Work out the finished part from the listing and answer in its coordinate system (mm). A direction names the side the tool comes from. Coordinates: 2 decimals unless noted, no trailing zeros. Order: outer loops, then holes, each group sorted by start corner. A loop starts at its lowest first (then second) coordinate and runs counter-clockwise, first axis right, second up. Notation, with made-up numbers: M -33,54 L 23,54 A34 cw 23,93 Z; hole C 47.5,80.25 d2. An arc over 180 degrees is marked long. Use a Markdown table: item, result. Add a question column.
from build123d import *

# Parameters (mm, degrees)
SKETCH1_W               = 25.4
SKETCH1_H               = 3.175
SKETCH1_W_2             = 1.5875
SKETCH1_H_2             = 1.5875
SKETCH1_W_3             = 7.9375
SKETCH1_H_3             = 2.38125
CUT_EXTRUDE1_DEPTH      = 27.940768363
CUT_EXTRUDE1_DEPTH_BACK = 27.940768363
SKETCH2_W               = 0.79375
SKETCH2_H               = 3.175
SKETCH2_R               = 1.5875
FILLET1_R               = 1.5875
CHAMFER1_SIZE           = 1.5875


with BuildPart() as part:
    # Sketch1 → Revolve1 (revolve)
    with BuildSketch(Plane.XY):
        with Locations((-12.7, 1.5875)):
            Rectangle(SKETCH1_W, SKETCH1_H)
        with Locations((-0.79375, 3.96875)):
            Rectangle(SKETCH1_W_2, SKETCH1_H_2)
        Polygon((0, 3.175), (0, 0), (2.38125, 0), (2.38125, 3.96875), (2.38125, 6.35), (0, 6.35), (0, 4.7625), align=None)
        with Locations((6.35, 5.159375)):
            Rectangle(SKETCH1_W_3, SKETCH1_H_3)
    revolve(axis=Axis((0, 0, 0), (-1, 0, 0)))

    # Sketch2 → Cut-Extrude1 (cut, two sides: drawn at the far end of the back side and taken through both)
    with BuildSketch(Plane(origin=(0, 0, 0), x_dir=(1, 0, 0), z_dir=(0, 1, 0)).offset(-CUT_EXTRUDE1_DEPTH_BACK)):
        with Locations((2.778125, 0)):
            Rectangle(SKETCH2_W, SKETCH2_H)
        with BuildLine():
            Line((3.175, -1.5875), (6.35, -1.5875))
            ThreePointArc((6.35, -1.5875), (4.7625, 0), (6.35, 1.5875))
            Line((6.35, 1.5875), (3.175, 1.5875))
            Line((3.175, 1.5875), (3.175, -1.5875))
        make_face()
        with Locations((6.35, 0)):
            Circle(SKETCH2_R)
        with BuildLine():
            Line((6.35, -1.5875), (10.31875, -1.5875))
            Line((10.31875, -1.5875), (10.31875, 1.5875))
            Line((10.31875, 1.5875), (6.35, 1.5875))
            ThreePointArc((6.35, 1.5875), (7.472532015, 1.122532015), (7.9375, 0))
            ThreePointArc((7.9375, 0), (7.472532015, -1.122532015), (6.35, -1.5875))
        make_face()
    extrude(amount=CUT_EXTRUDE1_DEPTH + CUT_EXTRUDE1_DEPTH_BACK, mode=Mode.SUBTRACT)

    # Fillet1
    fillet1_edges = [part.edges().sort_by_distance(p)[0] for p in [
        (2.38125, -4.89289026, -1.5875),
        (2.38125, 4.89289026, -1.5875),
        (2.38125, -4.89289026, 1.5875),
        (2.38125, 4.89289026, 1.5875),
    ]]
    fillet(fillet1_edges, radius=FILLET1_R - 0.0001)  # a hair under: the kernel refuses the full size

    # Chamfer1
    chamfer1_edges = [part.edges().sort_by_distance(p)[0] for p in [
        (10.31875, 0, 3.96875),
        (10.31875, 0, -3.96875),
    ]]
    chamfer(chamfer1_edges, length=CHAMFER1_SIZE)


solid = part.part
(1) Given P1, Ø6, axis at x = -10.5, y = 3.5, coming from the -Z side; P2, Ø2, axis at x = 8, y = -5, coming from the -Z side; P3, Ø1, axis at y = 2, z = -4.5, coming from the -X side; P4, Ø1.5, axis at x = -11, y = 4, coming from the -Z side, each flat-ended and moving along its own axis, determine where each tip first touches the part or whether it passes through.
(2) A cutting plane is placed at D-D on x = -12. Write down the section's boundary in (y, z) (3 decimals).
(3) The mould has two halves that part along Z. Classify faces 5 (the flat face through (0, 1, -5)), 6 (the cylindrical face through (2.859, 5.013, -1.135)), 7 (the cylindrical face through (-0.78, -3.78, 2.9)): pulls with the +Z half, pulls with the -Z half, needs draft (parallel to the pull), parting line crosses it, or undercut.
(4) Straight lines are drawn through the part: line 1 (X direction, y = -0.5, z = -3.5); line 2 (Z direction, x = 3, y = -1.75); line 3 (X direction, y = -2.75, z = 0.5). For each, find the intervals that lie inside material, in ascending order.
(5) A cutting plane is placed at C-C on z = -1. Write down the section's boundary in (x, y).
(6) A cutting plane is placed at A-A on x = 3.5. Write down the section's boundary in (y, z), plus the area to 3 significant figures.
(7) Which of the six approach directions +Z, -Z, +X, -X, +Y, -Y give full straight-line access (tool end or side, diameter ignored) to faces 1 (the flat face through (-25.4, 0, 0)), 2 (the cylindrical face through (-13.33, -0.69, 3.1)), 3 (the flat face through (7, 5, 1.588)), 4 (the cylindrical face through (5.601, 0.087, -3.968))?
From the geometry:
| question | item | result |
|---|---|---|
| 1 | P1 | stops at z = -3.14 |
| 1 | P2 | stops at z = -4.93 |
| 1 | P3 | stops at x = -1.59 |
| 1 | P4 | passes through |
| 2 | outline | C 0,0 d6.35 |
| 3 | face 5 | needs draft |
| 3 | face 6 | undercut |
| 3 | face 7 | parting line crosses it |
| 4 | line 1 | x = -1.59 to 2.38 |
| 4 | line 2 | z = -6.1 to -3.56, 3.56 to 6.1 |
| 4 | line 3 | x = -25.4 to 2.38 |
| 5 | outline | M -25.4,-3.01 L -1.59,-3.01 L -1.59,-4.66 L 0,-4.66 L 0,-6.27 L 2.74,-6.27 L 2.74,-3.84 L 2.38,-3.84 L 2.38,3.84 L 2.74,3.84 L 2.74,6.27 L 0,6.27 L 0,4.66 L -1.59,4.66 L -1.59,3.01 L -25.4,3.01 Z |
| 6 | outline | M -6.17,-1.52 A6.35 ccw 6.17,-1.52 L 3.67,-1.52 A3.97 cw -3.67,-1.52 Z; M -6.17,1.52 L -3.67,1.52 A3.97 cw 3.67,1.52 L 6.17,1.52 A6.35 ccw Z |
| 6 | area | 62.5 mm2 |
| 7 | face 1 | +Z, -Z, -X, +Y, -Y |
| 7 | face 2 | -X |
| 7 | face 3 | +X, +Y, -Y |
| 7 | face 4 | +X |
